Could you check a few things on this model? Use its own coordinates, in mm. A direction names the side the tool comes from. Round coordinates to 2 decimals unless told otherwise and drop trailing zeros. Write each loop counter-clockwise with the first axis right and the second up, starting at its lowest first coordinate (ties: lowest second). Pieces come first, ordered by that corner, then holes.
```python
from build123d import *

# Parameters (mm, degrees)
BOSS_EXTRUDE1_DEPTH  = 5.6
SHELL1_T             = -1.8
CUT_EXTRUDE1_REACH   = 72.916
SKETCH2_W            = 53.15
SKETCH2_H            = 3.8
SKETCH3_W            = 0.5
SKETCH3_H            = 0.75
CUT_EXTRUDE2_DEPTH   = 5.6
LPATTERN1_COUNT      = 5
LPATTERN1_PITCH      = 1.5
SKETCH4_R            = 3.45
SKETCH4_R_2          = 1.05
BOSS_EXTRUDE2_DEPTH  = 1.66
SKETCH5_R            = 1
BOSS_EXTRUDE3_DEPTH  = 2
CHAMFER1_SIZE        = 0.5
SKETCH6_R            = 2.5
CUT_EXTRUDE3_DEPTH   = 2
CUT_EXTRUDE4_DEPTH   = 1
LPATTERN2_COUNT      = 2
LPATTERN2_PITCH      = 39
MIRROR1_COPY_1_DEPTH = 1
SKETCH8_W            = 56.75
SKETCH8_H            = 10.5
CUT_EXTRUDE5_DEPTH   = 0.25
SKETCH9_W            = 3
SKETCH9_H            = 54.25
CUT_EXTRUDE6_DEPTH   = 0.1
SKETCH10_W           = 20
SKETCH10_H           = 3
CUT_EXTRUDE7_DEPTH   = 0.1
SKETCH11_W           = 3
SKETCH11_H           = 2.3
CUT_EXTRUDE8_DEPTH   = 0.1


with BuildPart() as part:
    # Sketch1 → Boss-Extrude1 (new body)
    with BuildSketch(Plane(origin=(0, 0, 0), x_dir=(1, 0, 0), z_dir=(0, 1, 0))):
        Polygon((23.375, 32.375), (-28.375, 32.375), (-28.375, -32.375), (28.375, -32.375), (28.375, 29.375), (23.375, 29.375), align=None)
    extrude(amount=BOSS_EXTRUDE1_DEPTH)

    # Shell1
    shell1_openings = [part.faces().sort_by_distance(p)[0] for p in [
        (-0.10605776, 5.6, 0.126552013),
    ]]
    offset(amount=SHELL1_T, openings=shell1_openings, kind=Kind.INTERSECTION)

    # Sketch2 → Cut-Extrude1 (cut, up to next)
    with BuildSketch(Plane.XY.offset(32.375), mode=Mode.PRIVATE) as cut_extrude1_sk1:
        with Locations((0, 3.7)):
            Rectangle(SKETCH2_W, SKETCH2_H)
    cut_extrude1_tool1 = extrude(cut_extrude1_sk1.sketch, amount=-CUT_EXTRUDE1_REACH, mode=Mode.PRIVATE) & part.part
    add(cut_extrude1_tool1.solids().sort_by_distance((0, 3.7, 32.375))[0], mode=Mode.SUBTRACT)

    # Sketch3 → Cut-Extrude2 (cut)
    with BuildSketch(Plane.XZ):
        with Locations((-28.125, -26.5)):
            Rectangle(SKETCH3_W, SKETCH3_H)
        with Locations((28.125, -26.5)):
            Rectangle(SKETCH3_W, SKETCH3_H)
    cut_extrude2 = extrude(amount=-CUT_EXTRUDE2_DEPTH, mode=Mode.SUBTRACT)

    # LPattern1: Cut-Extrude2 ×5
    with Locations(*[(0, 0, i * LPATTERN1_PITCH) for i in range(1, LPATTERN1_COUNT)]):
        add(cut_extrude2, mode=Mode.SUBTRACT)

    # Sketch4 → Boss-Extrude2 (add)
    with BuildSketch(Plane(origin=(0, 1.8, 0), x_dir=(1, 0, 0), z_dir=(0, 1, 0))):
        with Locations(Location((0, -15.425, 0), (0, 0, 90))):
            Circle(SKETCH4_R)
        with Locations(Location((0, -15.425, 0), (0, 0, 90))):
            Circle(SKETCH4_R_2, mode=Mode.SUBTRACT)
    extrude(amount=BOSS_EXTRUDE2_DEPTH)

    # Sketch5 → Boss-Extrude3 (add)
    with BuildSketch(Plane(origin=(0, 1.8, 0), x_dir=(1, 0, 0), z_dir=(0, 1, 0))):
        with Locations(Location((0, 9.375, 0), (0, 0, 90))):
            Circle(SKETCH5_R)
    extrude(amount=BOSS_EXTRUDE3_DEPTH)

    # Chamfer1
    chamfer1_edges = [part.edges().sort_by_distance(p)[0] for p in [
        (0, 3.46, 18.875),
        (0, 3.8, -8.375),
    ]]
    chamfer(chamfer1_edges, length=CHAMFER1_SIZE)

    # Sketch6 → Cut-Extrude3 (cut)
    with BuildSketch(Plane.XZ):
        with Locations(Location((0, 15.425, 0), (0, 0, 270))):
            Circle(SKETCH6_R)
    extrude(amount=-CUT_EXTRUDE3_DEPTH, mode=Mode.SUBTRACT)

    # Sketch7 → Cut-Extrude4 (cut)
    with BuildSketch(Plane.ZY.offset(-26.575)):
        with BuildLine():
            Line((15.375, 3.866149972), (15.375, 1.8))
            Line((15.375, 1.8), (21.375, 1.8))
            Line((21.375, 1.8), (21.375, 5.6))
            Line((21.375, 5.6), (18.375, 5.6))
            Line((18.375, 5.6), (18.375, 4.266149972))
            ThreePointArc((18.375, 4.266149972), (18.257842712, 3.98330726), (17.975, 3.866149972))
            Line((17.975, 3.866149972), (15.375, 3.866149972))
        make_face()
    cut_extrude4 = extrude(amount=-CUT_EXTRUDE4_DEPTH, mode=Mode.SUBTRACT)

    # LPattern2: Cut-Extrude4 ×2
    with Locations(*[(0, 0, -i * LPATTERN2_PITCH) for i in range(1, LPATTERN2_COUNT)]):
        add(cut_extrude4, mode=Mode.SUBTRACT)

    # Mirror1: Cut-Extrude4 across plane
    add(cut_extrude4.mirror(Plane(origin=(0, 0, 0), x_dir=(0, 0, 1), z_dir=(1, 0, 0))), mode=Mode.SUBTRACT)

    # Mirror1 copy 1 sketch → Mirror1 copy 1 (cut)
    with BuildSketch(Plane(origin=(-26.575, 0, -39), x_dir=(0, 0, 1), z_dir=(1, 0, 0))):
        with BuildLine():
            Line((15.375, -3.866149972), (15.375, -1.8))
            Line((15.375, -1.8), (21.375, -1.8))
            Line((21.375, -1.8), (21.375, -5.6))
            Line((21.375, -5.6), (18.375, -5.6))
            Line((18.375, -5.6), (18.375, -4.266149972))
            ThreePointArc((18.375, -4.266149972), (18.257842712, -3.98330726), (17.975, -3.866149972))
            Line((17.975, -3.866149972), (15.375, -3.866149972))
        make_face()
    extrude(amount=-MIRROR1_COPY_1_DEPTH, mode=Mode.SUBTRACT)

    # Sketch8 → Cut-Extrude5 (cut)
    with BuildSketch(Plane.XZ):
        with Locations((0, 27.125)):
            Rectangle(SKETCH8_W, SKETCH8_H)
    extrude(amount=-CUT_EXTRUDE5_DEPTH, mode=Mode.SUBTRACT)

    # Sketch9 → Cut-Extrude6 (cut)
    with BuildSketch(Plane.XZ):
        with Locations((14.875, -5.25)):
            Rectangle(SKETCH9_W, SKETCH9_H)
    cut_extrude6 = extrude(amount=-CUT_EXTRUDE6_DEPTH, mode=Mode.SUBTRACT)

    # Mirror2: Cut-Extrude6 across plane
    add(cut_extrude6.mirror(Plane(origin=(0, 0, 0), x_dir=(0, 0, 1), z_dir=(1, 0, 0))), mode=Mode.SUBTRACT)

    # Sketch10 → Cut-Extrude7 (cut)
    with BuildSketch(Plane.XZ):
        with Locations((0, -28.875)):
            Rectangle(SKETCH10_W, SKETCH10_H)
    extrude(amount=-CUT_EXTRUDE7_DEPTH, mode=Mode.SUBTRACT)

    # Sketch11 → Cut-Extrude8 (cut)
    with BuildSketch(Plane.XY.offset(-30.575)):
        with Locations((0, 2.95)):
            Rectangle(SKETCH11_W, SKETCH11_H)
    extrude(amount=-CUT_EXTRUDE8_DEPTH, mode=Mode.SUBTRACT)


solid = part.part
```
Q1. Imagine slicing it at A-A, the plane z = 26.5. Write out the boundary of the cut face in (x, y) (3 decimals).
Q2. On a 3-axis mill with a long thin cutter (end or side, diameter ignored), from which of +Z, -Z, +X, -X, +Y, -Y can I reach the whole of each face in a straight line? I mean faces 4 (the cylindrical face through (1.321, 2.372, 12.238)), 5 (the flat face through (-27.575, 3, 19)), 6 (the flat face through (26.575, 4, -25)), 7 (the flat face through (26, 3, -29.375)), 8 (the flat face through (0, 2, 14)). Say none if no direction works.
Q3. Imagine slicing it at B-B, the plane x = -5. Write out the boundary of the cut face in (y, z) (3 decimals).
Q4. I'm going to push flat-ended pins straight in: pin 1 Ø2 at (x, z) = (0, 5.5) entering from +Y; pin 2 Ø12 at (x, z) = (-2.5, 12) entering from +Y; pin 3 Ø0.9 at (x, z) = (-15, -16.5) entering from -Y. Where does each tip first touch, or does it pass through?
Q5. If I drill on L1, parallel to X at y = 4.5, z = 30 (3 decimals); L2, parallel to X at y = 2.65, z = -9 (3 decimals); L3, parallel to X at y = 2.9, z = -28 (3 decimals), over which ranges is the centre line in solid material (lowest first)?
Q6. We'd pull the mould along Y, two halves only. Please class faces 1 (the flat face through (-27.575, 3, -20)), 2 (the flat face through (23.375, 3, -31)), 3 (the flat face through (22, 0, -6)): pulls with the +Y half, pulls with the -Y half, needs draft (parallel to the pull), parting line crosses it, or undercut.
Q7. Imagine slicing it at C-C, the plane z = -18.5. Write out the boundary of the cut face in (x, y) (3 decimals), then the cut area to 3 significant figures.
Q8. Imagine slicing it at D-D, the plane x = -19.5. Write out the boundary of the cut face in (y, z) (3 decimals).
Results found:
1. outline: (-28.375, 0.25) - (28.375, 0.25) - (28.375, 5.6) - (26.575, 5.6) - (26.575, 1.8) - (-26.575, 1.8) - (-26.575, 5.6) - (-28.375, 5.6) - close
2. face 4: +Y
2. face 5: none
2. face 6: +Z, +Y
2. face 7: -Z, +X, +Y, -Y
2. face 8: -Y
3. outline: (0, -32.375) - (5.6, -32.375) - (5.6, -30.575) - (1.8, -30.575) - (1.8, 32.375) - (0.25, 32.375) - (0.25, 21.875) - (0, 21.875) - (0, -27.375) - (0.1, -27.375) - (0.1, -30.375) - (0, -30.375) - close
4. pin 1: stops at y = 1.8
4. pin 2: stops at y = 3.46
4. pin 3: stops at y = 0.1
5. L1: x = -28.375 to -26.575, 26.575 to 28.375
5. L2: x = -28.375 to -26.575, -0.927 to 0.927, 26.575 to 28.375
5. L3: x = -28.375 to -26.575, 21.575 to 28.375
6. face 1: undercut
6. face 2: needs draft
6. face 3: pulls with the -Y half
7. outline: (-28.375, 0) - (-16.375, 0) - (-16.375, 0.1) - (-13.375, 0.1) - (-13.375, 0) - (13.375, 0) - (13.375, 0.1) - (16.375, 0.1) - (16.375, 0) - (28.375, 0) - (28.375, 5.6) - (27.575, 5.6) - (27.575, 1.8) - (-27.575, 1.8) - (-27.575, 5.6) - (-28.375, 5.6) - close
7. area: 108 mm2
8. outline: (0, -32.375) - (5.6, -32.375) - (5.6, -30.575) - (1.8, -30.575) - (1.8, 32.375) - (0.25, 32.375) - (0.25, 21.875) - (0, 21.875) - close
